```python
from build123d import *

# Parameters (mm, degrees)
SKETCH1_R                 = 25
BOSS_EXTRUDE1_DEPTH       = 4.3
BOSS_EXTRUDE2_START       = 4.3
BOSS_EXTRUDE2_OUTLINE_R   = 25
BOSS_EXTRUDE2_DEPTH       = 2
BOSS_EXTRUDE2_START_2     = -8
BOSS_EXTRUDE2_2_OUTLINE_W = 53
BOSS_EXTRUDE2_2_OUTLINE_H = 52
BOSS_EXTRUDE2_2_DEPTH     = 2.704234919
CUT_EXTRUDE1_REACH        = 37.912
SKETCH3_R                 = 1.55
CUT_EXTRUDE2_REACH        = 37.616
SKETCH4_R                 = 3.25


with BuildPart() as part:
    # Sketch1 → Boss-Extrude1 (new body)
    with BuildSketch(Plane(origin=(0, 0, 0), x_dir=(1, 0, 0), z_dir=(0, 1, 0))):
        with Locations(Location((0, 0, 0), (0, 0, 90))):
            Circle(SKETCH1_R)
    extrude(amount=BOSS_EXTRUDE1_DEPTH)

    # Boss-Extrude2: read off the stored shape, not the designer's step
    # Boss-Extrude2 outline → Boss-Extrude2 (add)
    with BuildSketch(Plane(origin=(0, 0, 0), x_dir=(1, 0, 0), z_dir=(0, 1, 0)).offset(BOSS_EXTRUDE2_START)):
        Circle(BOSS_EXTRUDE2_OUTLINE_R)
    extrude(amount=BOSS_EXTRUDE2_DEPTH)

    # Boss-Extrude2 2 outline → Boss-Extrude2 2 (cut)
    with BuildSketch(Plane(origin=(0, 0, 0), x_dir=(0.9992009587217894, 0.03996803834887162, 0), z_dir=(0.03996803834887162, -0.9992009587217895, 0)).offset(BOSS_EXTRUDE2_START_2)):
        with Locations((0.5, 0)):
            Rectangle(BOSS_EXTRUDE2_2_OUTLINE_W, BOSS_EXTRUDE2_2_OUTLINE_H)
    extrude(amount=BOSS_EXTRUDE2_2_DEPTH, mode=Mode.SUBTRACT)

    # Cut-Extrude1: up to this plane
    cut_extrude1_end = Plane(origin=(-25, 4.3, 25.001), z_dir=(0.03996803834887159, -0.9992009587217895, 0))
    # Sketch3 → Cut-Extrude1 (cut, up to the surface)
    with BuildSketch(Plane(origin=(0, 0, 0), x_dir=(1, 0, 0), z_dir=(0, 1, 0)), mode=Mode.PRIVATE) as cut_extrude1_sk1:
        with Locations(Location((-15.244012286, -6.314276634, 0), (0, 0, 180))):
            Circle(SKETCH3_R)
    cut_extrude1_tool1 = split(extrude(cut_extrude1_sk1.sketch, amount=CUT_EXTRUDE1_REACH, mode=Mode.PRIVATE), bisect_by=cut_extrude1_end, keep=Keep.BOTH, mode=Mode.PRIVATE)
    add(cut_extrude1_tool1.solids().sort_by_distance((-15.244012, 0, 6.314277))[0], mode=Mode.SUBTRACT)
    # Sketch3 → Cut-Extrude1 (cut, up to the surface)
    with BuildSketch(Plane(origin=(0, 0, 0), x_dir=(1, 0, 0), z_dir=(0, 1, 0)), mode=Mode.PRIVATE) as cut_extrude1_sk2:
        with Locations(Location((2.153682172, 16.358840213, 0), (0, 0, 180))):
            Circle(SKETCH3_R)
    cut_extrude1_tool2 = split(extrude(cut_extrude1_sk2.sketch, amount=CUT_EXTRUDE1_REACH, mode=Mode.PRIVATE), bisect_by=cut_extrude1_end, keep=Keep.BOTH, mode=Mode.PRIVATE)
    add(cut_extrude1_tool2.solids().sort_by_distance((2.153682, 0, -16.35884))[0], mode=Mode.SUBTRACT)
    # Sketch3 → Cut-Extrude1 (cut, up to the surface)
    with BuildSketch(Plane(origin=(0, 0, 0), x_dir=(1, 0, 0), z_dir=(0, 1, 0)), mode=Mode.PRIVATE) as cut_extrude1_sk3:
        with Locations(Location((13.090330115, -10.044563579, 0), (0, 0, 180))):
            Circle(SKETCH3_R)
    cut_extrude1_tool3 = split(extrude(cut_extrude1_sk3.sketch, amount=CUT_EXTRUDE1_REACH, mode=Mode.PRIVATE), bisect_by=cut_extrude1_end, keep=Keep.BOTH, mode=Mode.PRIVATE)
    add(cut_extrude1_tool3.solids().sort_by_distance((13.09033, 0, 10.044564))[0], mode=Mode.SUBTRACT)

    # Cut-Extrude2: up to this plane
    cut_extrude2_end = Plane(origin=(-25, 4.3, 25.001), z_dir=(0.03996803834887159, -0.9992009587217895, 0))
    # Sketch4 → Cut-Extrude2 (cut, up to the surface)
    with BuildSketch(Plane(origin=(0, 2, 0), x_dir=(-1, 0, 0), z_dir=(0, -1, 0)), mode=Mode.PRIVATE) as cut_extrude2_sk1:
        with Locations(Location((-2.153682172, 16.358840213, 0), (0, 0, 90))):
            Circle(SKETCH4_R)
    cut_extrude2_tool1 = split(extrude(cut_extrude2_sk1.sketch, amount=-CUT_EXTRUDE2_REACH, mode=Mode.PRIVATE), bisect_by=cut_extrude2_end, keep=Keep.BOTH, mode=Mode.PRIVATE)
    add(cut_extrude2_tool1.solids().sort_by_distance((2.153682, 2, -16.35884))[0], mode=Mode.SUBTRACT)
    # Sketch4 → Cut-Extrude2 (cut, up to the surface)
    with BuildSketch(Plane(origin=(0, 2, 0), x_dir=(-1, 0, 0), z_dir=(0, -1, 0)), mode=Mode.PRIVATE) as cut_extrude2_sk2:
        with Locations(Location((15.244012286, -6.314276634, 0), (0, 0, 90))):
            Circle(SKETCH4_R)
    cut_extrude2_tool2 = split(extrude(cut_extrude2_sk2.sketch, amount=-CUT_EXTRUDE2_REACH, mode=Mode.PRIVATE), bisect_by=cut_extrude2_end, keep=Keep.BOTH, mode=Mode.PRIVATE)
    add(cut_extrude2_tool2.solids().sort_by_distance((-15.244012, 2, 6.314277))[0], mode=Mode.SUBTRACT)
    # Sketch4 → Cut-Extrude2 (cut, up to the surface)
    with BuildSketch(Plane(origin=(0, 2, 0), x_dir=(-1, 0, 0), z_dir=(0, -1, 0)), mode=Mode.PRIVATE) as cut_extrude2_sk3:
        with Locations(Location((-13.090330115, -10.044563579, 0), (0, 0, 90))):
            Circle(SKETCH4_R)
    cut_extrude2_tool3 = split(extrude(cut_extrude2_sk3.sketch, amount=-CUT_EXTRUDE2_REACH, mode=Mode.PRIVATE), bisect_by=cut_extrude2_end, keep=Keep.BOTH, mode=Mode.PRIVATE)
    add(cut_extrude2_tool3.solids().sort_by_distance((13.09033, 2, 10.044564))[0], mode=Mode.SUBTRACT)


solid = part.part
```
Here's how the part is built. I have some questions about the finished solid (model axes, mm). A direction names the side the tool comes from. Coordinates: 2 decimals unless noted, no trailing zeros. Order: outer loops, then holes, each group sorted by start corner. A loop starts at its lowest first (then second) coordinate and runs counter-clockwise, first axis right, second up. Notation, with made-up numbers: (9, 47.25) -> (17, 47.25) arc R25 cw to (17, 73.25) -> close; hole circle Ø11 at (-11.5, -32). An arc over 180 degrees is marked (long way). Return JSON: item names as keys, results as strings.
1) Thinking about a two-plate mould opening in Z: for faces 3 (the cylindrical face through (23.204, 4.506, -9.304)), 4 (the flat face through (-0.35, 5.286, 0.35)), 5 (the cylindrical face through (16.313, 3.962, 10.468)), which applies, +Z half, -Z half, draft (parallel to the pull), parting line (faces both ways), or undercut?
Conclusion:
{"face 3": "parting line", "face 4": "draft", "face 5": "undercut"}
2) If I drill on probe 1 along X at (y, z) = (3.25, 9); probe 2 along Z at (x, y) = (12.5, 0.75); probe 3 along X at (y, z) = (1.5, 21.5), over which ranges is the centre line in solid material (lowest first)?
Conclusion:
{"probe 1": "x = -23.32 to -17.07, -13.41 to 10.01, 16.17 to 23.32", "probe 2": "z = -21.65 to 8.61, 11.48 to 21.65", "probe 3": "x = -12.76 to 12.76"}
3) I'm going to push flat-ended pins straight in: P1, Ø5, axis at x = -14.5, z = 5, coming from the +Y side; P2, Ø2, axis at x = 13.5, z = 11, coming from the +Y side; P3, Ø1.5, axis at y = 3, z = 15.5, coming from the +X side. Where does each tip first touch, or does it pass through?
Conclusion:
{"P1": "stops at y = 4.82", "P2": "stops at y = 2", "P3": "stops at x = 20.19"}
4) On a 3-axis mill with a long thin cutter (end or side, diameter ignored), from which of +Z, -Z, +X, -X, +Y, -Y can I reach the whole of each face in a straight line? I mean faces 1 (the cylindrical face through (12.257, 0.986, 11.352)), 2 (the cylindrical face through (4.9, 3.7, -18.1)). Say none if no direction works.
Conclusion:
{"face 1": "+Y, -Y", "face 2": "+Y"}
5) If we section it at B-B on z = 0: List the corners of the cut face in (x, y) for me.
Conclusion:
{"outline": "(-25, 0) -> (25, 0) -> (25, 6.3) -> (-25, 4.3) -> close"}
6) If we section it at A-A on x = 0: List the corners of the cut face in (y, z) for me.
Conclusion:
{"outline": "(0, -25) -> (5.3, -25) -> (5.3, -18.79) -> (2, -18.79) -> (2, -13.92) -> (5.3, -13.92) -> (5.3, 25) -> (0, 25) -> close"}
7) If we section it at D-D on z = -7.5: List the corners of the cut face in (x, y) for me.
Conclusion:
{"outline": "(-23.85, 0) -> (23.85, 0) -> (23.85, 6.25) -> (-23.85, 4.35) -> close"}
8) If we section it at C-C on y = 3: List the corners of the cut face in (x, z) for me.
Conclusion:
{"outline": "circle Ø50 at (0, 0); hole circle Ø6.5 at (-15.24, 6.31); hole circle Ø6.5 at (2.15, -16.36); hole circle Ø6.5 at (13.09, 10.04)"}
